Autodesk Inventor part; units mm, degrees
ref_plane "YZ Plane" through (0, 0, 0) normal (1, 0, 0) x (0, 1, 0)
ref_plane "XZ Plane" through (0, 0, 0) normal (0, 1, 0) x (-1, 0, 0)
ref_plane "XY Plane" through (0, 0, 0) normal (0, 0, 1) x (1, 0, 0)
sketch "Sketch1" plane through (0, 0, 0) normal (0, 1, 0) x (-1, 0, 0)
  line L0 (0, 0) -> (25.4, 0)
  line L1 (25.4, 0) -> (25.4, 25.4)
  line L2 (25.4, 25.4) -> (0, 25.4)
  line L3 (0, 25.4) -> (0, 0)
  dimension "d0" = 25.4
  dimension "d1" = 25.4
extrude "Extrusion1" add sketch "Sketch1" along normal blind 8.89
sketch "Sketch2" plane through (0, 8.89, 0) normal (0, 1, 0) x (1, 0, 0)
  circle A0 centre (-12.7, -12.7) radius 9.525
  point P0 (-25.4, 0)
  dimension "d4" = 19.05
  dimension "d5" = 12.7
  dimension "d6" = 12.7
extrude "Extrusion2" cut sketch "Sketch2" against normal blind 7.1437
sketch "Sketch3" plane through (-12.7, 1.7463, 12.7) normal (0, 1, 0) x (1, 0, 0)
  circle A0 centre (0, 0) radius 9.525
  circle A1 centre (0, 0) radius 3.175
  circle A2 centre (0, 0) radius 6.35
  point P0 (12.7, 12.7)
  dimension "d9" = 6.35
  dimension "d12" = 3.175
  dimension "d13" = 3.175
extrude "Extrusion3" cut sketch "Sketch3" against normal through all contours A1 | A2
mirror "Mirror1" about plane through (-12.7, 0, 12.7) normal (0, -1, 0)
equation "\"d12\" = d13"
properties part number "acmeBearingBlock"
CAD build for the part. Positions are in the model's coordinates, mm. A direction names the side the tool comes from. Give positions to 0.01 mm unless a question says otherwise; leave off trailing zeros. Order: outer loops, then holes, each group sorted by start corner. A loop starts at its lowest first (then second) coordinate and runs counter-clockwise, first axis right, second up. Notation, with made-up numbers: (28.25, 38.5) -> (55.25, 38.5) arc R7 cw to (55.25, 46.5) -> close; hole circle Ø11 at (52.25, 22). An arc over 180 degrees is marked (long way). Return JSON: item names as keys, results as strings.
Q1. Mould opens along Z. For faces 4 (the face through (-20.259, -5.368, 6.904)), 5 (the face through (-25.4, 0, 13)), 6 (the face through (-13, 0, 0)) say: pulls with the +Z half, pulls with the -Z half, needs draft (parallel to the pull), parting line crosses it, or undercut.
Working result:
{"face 4": "undercut", "face 5": "needs draft", "face 6": "pulls with the -Z half"}
Q2. Saw through at B-B (x = -12.7). Write the cut outline in (y, z) (3 decimals), then the cut area to 3 significant figures.
Working result:
{"outline": "(-8.89, 0) -> (8.89, 0) -> (8.89, 3.175) -> (1.746, 3.175) -> (1.746, 6.35) -> (-1.746, 6.35) -> (-1.746, 3.175) -> (-8.89, 3.175) -> close; (-8.89, 22.225) -> (-1.746, 22.225) -> (-1.746, 19.05) -> (1.746, 19.05) -> (1.746, 22.225) -> (8.89, 22.225) -> (8.89, 25.4) -> (-8.89, 25.4) -> close", "area": "135 mm²"}
Q3. Saw through at D-D (z = 21.5). Write the cut outline in (x, y).
Working result:
{"outline": "(-25.4, -8.89) -> (-16.34, -8.89) -> (-16.34, -1.75) -> (-9.06, -1.75) -> (-9.06, -8.89) -> (0, -8.89) -> (0, 8.89) -> (-9.06, 8.89) -> (-9.06, 1.75) -> (-16.34, 1.75) -> (-16.34, 8.89) -> (-25.4, 8.89) -> close"}
Q4. Drill centre lines: line 1 (Z direction, x = -13, y = 3.5); line 2 (X direction, y = -6.75, z = 12.7) (3 decimals); line 3 (X direction, y = -0.6, z = 12.7). Where is each one in solid material? Low to high.
Working result:
{"line 1": "0 to 3.18, 22.22 to 25.4", "line 2": "-25.4 to -22.225, -3.175 to 0", "line 3": "-25.4 to -19.05, -6.35 to 0"}
Q5. Saw through at A-A (z = 12.7). Write the cut outline in (x, y) (3 decimals), then the cut area to 3 significant figures.
Working result:
{"outline": "(-25.4, -8.89) -> (-22.225, -8.89) -> (-22.225, -1.746) -> (-19.05, -1.746) -> (-19.05, 1.746) -> (-22.225, 1.746) -> (-22.225, 8.89) -> (-25.4, 8.89) -> close; (-6.35, -1.746) -> (-3.175, -1.746) -> (-3.175, -8.89) -> (0, -8.89) -> (0, 8.89) -> (-3.175, 8.89) -> (-3.175, 1.746) -> (-6.35, 1.746) -> close", "area": "135 mm²"}
Q6. Which spindle directions (+Z, -Z, +X, -X, +Y, -Y) get a long thin tool onto all of the face, cutting with end or side? Do faces 1 (the face through (-15, -1.746, 19)), 2 (the face through (-22.216, 5.368, 12.281)), 3 (the face through (-18, 8.89, 4)). Say none if no direction does.
Working result:
{"face 1": "-Y", "face 2": "+Y", "face 3": "+Z, -Z, +X, -X, +Y"}
Q7. Flat gauge pins, fed straight in: pin 1 (15 mm diameter, centred on x = -12.7, z = 12.7, fed in from -Y); pin 2 (11.5 mm diameter, centred on x = -12.7, z = 12.7, fed in from -Y). Where does each tip first touch, or does it go through?
Working result:
{"pin 1": "y = -1.75", "pin 2": "through"}
Q8. Saw through at C-C (y = 2.5). Write the cut outline in (x, z) (3 decimals), then the cut area to 3 significant figures.
Working result:
{"outline": "(-25.4, 0) -> (0, 0) -> (0, 25.4) -> (-25.4, 25.4) -> close; hole circle Ø19.05 at (-12.7, 12.7)", "area": "360 mm²"}
